Part model, mm, in its own coordinate system. Face numbers are marked on the shaded views. Give positions to 0.01 mm unless a question says otherwise; leave off trailing zeros. Order: outer loops, then holes, each group sorted by start corner. A loop starts at its lowest first (then second) coordinate and runs counter-clockwise, first axis right, second up. Notation, with made-up numbers: (64, 47.25) - (106, 47.25) arc R16 cw to (106, 64.25) - close; hole circle Ø6 at (83.5, 26). An arc over 180 degrees is marked (long way). One line per item, written item: value.
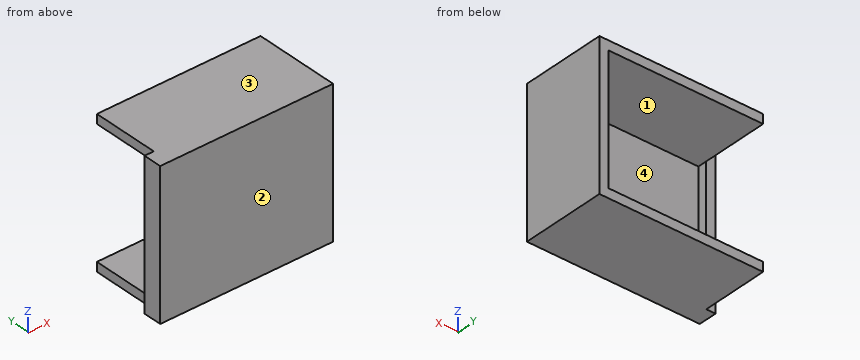
Autodesk Inventor part; units mm, degrees
ref_plane "YZ Plane" through (0, 0, 0) normal (1, 0, 0) x (0, 1, 0)
ref_plane "XZ Plane" through (0, 0, 0) normal (0, 1, 0) x (-1, 0, 0)
ref_plane "XY Plane" through (0, 0, 0) normal (0, 0, 1) x (1, 0, 0)
sketch "Sketch1" plane through (0, 0, 0) normal (0, 1, 0) x (-1, 0, 0)
  line L0 (0, 0) -> (67, 0)
  line L1 (67, 0) -> (67, -55)
  line L2 (67, -55) -> (0, -55)
  line L3 (0, -55) -> (0, 0)
  line L4 (-4, -59) -> (71, -59)
  line L5 (71, -59) -> (71, 4)
  line L6 (71, 4) -> (-4, 4)
  line L7 (-4, 4) -> (-4, -59)
  line L8 (67, 4) -> (67, -59)
  dimension "d0" = 67
  dimension "d1" = 55
  dimension "d2" = 4
extrude "Extrusion1" add sketch "Sketch1" along normal blind 33 contours L3 L2 L8 L4 L7 L6 L0
extrude "Extrusion2" add sketch "Sketch1" against normal blind 4
extrude "Extrusion3" add sketch "Sketch1" along normal blind 4 contours L8 L6 L5 L4 L1
properties part number "Z Fold Jig"
1) Two-plate mould, pull along Z, no slides. Class the marked faces 1, 2, 3 and 4: pulls with the +Z half, pulls with the -Z half, needs draft (parallel to the pull), parting line crosses it, or undercut.
Answer:
face 1: undercut
face 2: needs draft
face 3: pulls with the +Z half
face 4: undercut
2) Slice it at A-A on z = -1. Write the cut outline in (x, y), then the cut area to 3 significant figures.
Answer:
outline: (-71, -4) - (4, -4) - (4, 33) - (0, 33) - (0, 0) - (-67, 0) - (-67, 4) - (-71, 4) - close
area: 448 mm2
3) Drop flat-ended pins along their axis: P1, Ø1.5, axis at x = -51.5, z = -14.5, coming from the +Y side; P2, Ø1.5, axis at y = 29, z = -6.5, coming from the -X side; P3, Ø3, axis at y = 12, z = -57.5, coming from the -X side. Give the stop position or say it passes through.
Answer:
P1: stops at y = 0
P2: stops at x = 0
P3: stops at x = -67
4) Slice it at B-B on y = 13.5. Write the cut outline in (x, z).
Answer:
outline: (-67, -59) - (4, -59) - (4, 4) - (-67, 4) - (-67, 0) - (0, 0) - (0, -55) - (-67, -55) - close
5) Wall check: line 1 along Z through (x, y) = (-62.5, 15); line 2 along X through (y, z) = (1.5, -47); line 3 along X through (y, z) = (23, -12). Give the ranges that are in metal, low to high. Write a range as [from, to].
Answer:
line 1: z = [-59, -55], [0, 4]
line 2: x = [-71, -67], [0, 4]
line 3: x = [0, 4]
